Work out the finished part from the listing and answer in its coordinate system (mm). A direction names the side the tool comes from. Round coordinates to 2 decimals unless told otherwise and drop trailing zeros. Write each loop counter-clockwise with the first axis right and the second up, starting at its lowest first coordinate (ties: lowest second). Pieces come first, ordered by that corner, then holes.
1. Flat-ended cylindrical pins translate along their axes: pin 1 Ø1.6 at (x, y) = (16.5, -9.5) entering from +Z; pin 2 Ø11 at (x, y) = (10, -10) entering from -Z. Find the tip coordinate at first contact, or state that the pin passes through.
2. A tool of negligible diameter and unlimited length cuts with its end or side. For faces 1 (the face through (11, -8, 4)), 2 (the face through (16, -10, 5)), 3 (the face through (2, -19, 4)), from which of +Z, -Z, +X, -X, +Y, -Y can it reach the whole face along a straight path? Write none if from no direction.
3. Find section C-C (z = 7.25). Write down the section's boundary in (x, y).
4. Determine the mould class of faces 4 (the face through (10, -20, 4)), 5 (the face through (20, -10, 4)), 6 (the face through (4, -9, 7)) for opening direction Y: pulls with the +Y half, pulls with the -Y half, needs draft (parallel to the pull), parting line crosses it, or undercut.
5. Find section A-A (y = -18). Write down the section's boundary in (x, z).
6. Straight lines are drawn through the part: probe 1 along Y at (x, z) = (2, 6.75); probe 2 along Y at (x, z) = (4, 5.85); probe 3 along Y at (x, z) = (10, 7.55). For each, find the intervals that lie inside material, in ascending order.
7. Find section B-B (x = 10). Write down the section's boundary in (y, z).
8. Find section D-D (x = 18). Write down the section's boundary in (y, z), and give its area (3 significant figures).
```python
from build123d import *

# Parameters (mm, degrees)
F0_W     = 20
F0_H     = 20
F0_R     = 1
F0_R_2   = 8.5
F0_R_3   = 7
F0_R_4   = 6.5
F0_R_5   = 1.25
F0_R_6   = 2
F1_DEPTH = 8
F2_R     = 3.5
F2_R_2   = 2
F3_DEPTH = 2
F4_SIZE  = 0.1
F5_DEPTH = 4
F6_R     = 1
F7_DEPTH = 3


with BuildPart() as f1:
    # F0 (on Top) → F1 (new body)
    with BuildSketch(Plane.XY):
        with Locations((10, -10)):
            Rectangle(F0_W, F0_H)
        with Locations((2, -18)):
            Circle(F0_R, mode=Mode.SUBTRACT)
        with Locations((18, -18)):
            Circle(F0_R, mode=Mode.SUBTRACT)
        with Locations((2, -2)):
            Circle(F0_R, mode=Mode.SUBTRACT)
        with Locations((10, -10)):
            Circle(F0_R_2, mode=Mode.SUBTRACT)
        with Locations((18, -2)):
            Circle(F0_R, mode=Mode.SUBTRACT)
        with Locations((10, -10)):
            Circle(F0_R_2)
        with Locations((10, -10)):
            Circle(F0_R_3, mode=Mode.SUBTRACT)
        with Locations((10, -10)):
            Circle(F0_R_3)
        with Locations((10, -10)):
            Circle(F0_R_4, mode=Mode.SUBTRACT)
        with Locations((10, -10)):
            Circle(F0_R_4)
        with BuildLine():
            ThreePointArc((11.25, -14.25), (9.1161165153, -15.1338834682), (10.0000000233, -13))
            ThreePointArc((10.0000000233, -13), (10.8838834847, -13.3661165318), (11.25, -14.25))
        make_face(mode=Mode.SUBTRACT)
        with Locations((5.75, -10)):
            Circle(F0_R_5, mode=Mode.SUBTRACT)
        with BuildLine():
            ThreePointArc((10, -7), (12.1213203436, -7.8786796564), (13, -10))
            ThreePointArc((13, -10), (12.1213203518, -12.1213203353), (10.0000000233, -13))
            ThreePointArc((10.0000000233, -13), (7.8786796647, -12.1213203518), (7, -10))
            ThreePointArc((7, -10), (7.8786796564, -7.8786796564), (10, -7))
        make_face(mode=Mode.SUBTRACT)
        with BuildLine():
            ThreePointArc((15.5, -10), (14.25, -11.25), (13, -10))
            ThreePointArc((13, -10), (14.25, -8.75), (15.5, -10))
        make_face(mode=Mode.SUBTRACT)
        with BuildLine():
            ThreePointArc((11.25, -5.75), (10.8838834765, -6.6338834765), (10, -7))
            ThreePointArc((10, -7), (9.1161165235, -4.8661165235), (11.25, -5.75))
        make_face(mode=Mode.SUBTRACT)
        with BuildLine():
            ThreePointArc((10.0000000233, -13), (12.1213203518, -12.1213203353), (13, -10))
            ThreePointArc((13, -10), (12.1213203436, -7.8786796564), (10, -7))
            ThreePointArc((10, -7), (7.8786796564, -7.8786796564), (7, -10))
            ThreePointArc((7, -10), (7.8786796647, -12.1213203518), (10.0000000233, -13))
        make_face()
        with Locations((10, -10)):
            Circle(F0_R_6, mode=Mode.SUBTRACT)
        with BuildLine():
            ThreePointArc((15.5, -10), (14.25, -8.75), (13, -10))
            ThreePointArc((13, -10), (14.25, -11.25), (15.5, -10))
        make_face()
        with BuildLine():
            ThreePointArc((11.25, -5.75), (9.1161165235, -4.8661165235), (10, -7))
            ThreePointArc((10, -7), (10.8838834765, -6.6338834765), (11.25, -5.75))
        make_face()
        with Locations((5.75, -10)):
            Circle(F0_R_5)
        with BuildLine():
            ThreePointArc((11.25, -14.25), (10.8838834847, -13.3661165318), (10.0000000233, -13))
            ThreePointArc((10.0000000233, -13), (9.1161165153, -15.1338834682), (11.25, -14.25))
        make_face()
    extrude(amount=F1_DEPTH)

    # F2 (on face) → F3 (cut)
    with BuildSketch(Plane.XY.offset(8)):
        with Locations((10, -10)):
            Circle(F2_R)
        with Locations((10, -10)):
            Circle(F2_R_2, mode=Mode.SUBTRACT)
    extrude(amount=-F3_DEPTH, mode=Mode.SUBTRACT)

    # F4
    f4_edges = [f1.edges().sort_by_distance(p)[0] for p in [
        (10, 0, 8),
        (20, -10, 8),
        (0, -10, 8),
        (10, -20, 8),
        (1, -18, 8),
        (17, -18, 8),
        (1, -2, 8),
        (6.5, -10, 8),
        (17, -2, 8),
        (20, -20, 4),
        (20, 0, 4),
        (0, -20, 4),
        (0, 0, 4),
        (8, -10, 6),
    ]]
    chamfer(f4_edges, length=F4_SIZE)

    # F0 (on Top) → F5 (cut)
    with BuildSketch(Plane.XY):
        with Locations((10, -10)):
            Circle(F0_R_4)
        with BuildLine():
            ThreePointArc((11.25, -14.25), (9.1161165153, -15.1338834682), (10.0000000233, -13))
            ThreePointArc((10.0000000233, -13), (10.8838834847, -13.3661165318), (11.25, -14.25))
        make_face(mode=Mode.SUBTRACT)
        with Locations((5.75, -10)):
            Circle(F0_R_5, mode=Mode.SUBTRACT)
        with BuildLine():
            ThreePointArc((10, -7), (12.1213203436, -7.8786796564), (13, -10))
            ThreePointArc((13, -10), (12.1213203518, -12.1213203353), (10.0000000233, -13))
            ThreePointArc((10.0000000233, -13), (7.8786796647, -12.1213203518), (7, -10))
            ThreePointArc((7, -10), (7.8786796564, -7.8786796564), (10, -7))
        make_face(mode=Mode.SUBTRACT)
        with BuildLine():
            ThreePointArc((15.5, -10), (14.25, -11.25), (13, -10))
            ThreePointArc((13, -10), (14.25, -8.75), (15.5, -10))
        make_face(mode=Mode.SUBTRACT)
        with BuildLine():
            ThreePointArc((11.25, -5.75), (10.8838834765, -6.6338834765), (10, -7))
            ThreePointArc((10, -7), (9.1161165235, -4.8661165235), (11.25, -5.75))
        make_face(mode=Mode.SUBTRACT)
        with BuildLine():
            ThreePointArc((10.0000000233, -13), (12.1213203518, -12.1213203353), (13, -10))
            ThreePointArc((13, -10), (12.1213203436, -7.8786796564), (10, -7))
            ThreePointArc((10, -7), (7.8786796564, -7.8786796564), (7, -10))
            ThreePointArc((7, -10), (7.8786796647, -12.1213203518), (10.0000000233, -13))
        make_face()
        with Locations((10, -10)):
            Circle(F0_R_6, mode=Mode.SUBTRACT)
        with BuildLine():
            ThreePointArc((15.5, -10), (14.25, -8.75), (13, -10))
            ThreePointArc((13, -10), (14.25, -11.25), (15.5, -10))
        make_face()
        with BuildLine():
            ThreePointArc((11.25, -14.25), (10.8838834847, -13.3661165318), (10.0000000233, -13))
            ThreePointArc((10.0000000233, -13), (9.1161165153, -15.1338834682), (11.25, -14.25))
        make_face()
        with Locations((5.75, -10)):
            Circle(F0_R_5)
        with BuildLine():
            ThreePointArc((11.25, -5.75), (9.1161165235, -4.8661165235), (10, -7))
            ThreePointArc((10, -7), (10.8838834765, -6.6338834765), (11.25, -5.75))
        make_face()
    extrude(amount=F5_DEPTH, mode=Mode.SUBTRACT)

    # F6 (on face) → F7 (cut)
    with BuildSketch(Plane.XY.offset(8)):
        with Locations((4, -10)):
            Circle(F6_R)
        with Locations((16, -10)):
            Circle(F6_R)
    extrude(amount=-F7_DEPTH, mode=Mode.SUBTRACT)


solid = f1.part
```
Worked answers:
1. pin 1: stops at z = 8
1. pin 2: stops at z = 4
2. face 1: -Z
2. face 2: +Z
2. face 3: +Z, -Z
3. outline: (0, -19.9) - (0.1, -20) - (19.9, -20) - (20, -19.9) - (20, -0.1) - (19.9, 0) - (0.1, 0) - (0, -0.1) - close; hole circle Ø2 at (2, -18); hole circle Ø2 at (2, -2); hole circle Ø2 at (4, -10); hole circle Ø7 at (10, -10); hole circle Ø2 at (16, -10); hole circle Ø2 at (18, -18); hole circle Ø2 at (18, -2)
4. face 4: pulls with the -Y half
4. face 5: needs draft
4. face 6: undercut
5. outline: (0, 0) - (1, 0) - (1, 7.9) - (0.9, 8) - (0.1, 8) - (0, 7.9) - close; (3, 0) - (17, 0) - (17, 7.9) - (16.9, 8) - (3.1, 8) - (3, 7.9) - close; (19, 0) - (20, 0) - (20, 7.9) - (19.9, 8) - (19.1, 8) - (19, 7.9) - close
6. probe 1: y = -20 to -19, -17 to -3, -1 to 0
6. probe 2: y = -20 to -11, -9 to 0
6. probe 3: y = -20 to -13.5, -6.5 to 0
7. outline: (-20, 0) - (-16.5, 0) - (-16.5, 4) - (-12, 4) - (-12, 5.9) - (-12.1, 6) - (-13.5, 6) - (-13.5, 7.9) - (-13.6, 8) - (-19.9, 8) - (-20, 7.9) - close; (-8, 4) - (-3.5, 4) - (-3.5, 0) - (0, 0) - (0, 7.9) - (-0.1, 8) - (-6.4, 8) - (-6.5, 7.9) - (-6.5, 6) - (-7.9, 6) - (-8, 5.9) - close
8. outline: (-20, 0) - (-19, 0) - (-19, 7.9) - (-19.1, 8) - (-19.9, 8) - (-20, 7.9) - close; (-17, 0) - (-3, 0) - (-3, 7.9) - (-3.1, 8) - (-16.9, 8) - (-17, 7.9) - close; (-1, 0) - (0, 0) - (0, 7.9) - (-0.1, 8) - (-0.9, 8) - (-1, 7.9) - close
8. area: 128 mm2
